```python
from build123d import *

# Parameters (mm, degrees)
SKETCH1_W           = 104
SKETCH1_H           = 104
BOSS_EXTRUDE1_DEPTH = 57.5
BOSS_EXTRUDE1_TAPER = 23
SKETCH2_R           = 25
CUT_EXTRUDE1_DEPTH  = 187.700294763
FILLET1_R           = 15
SKETCH3_R           = 35
CUT_EXTRUDE2_DEPTH  = 10
CUT_EXTRUDE3_START  = -10
SKETCH5_R           = 35
CUT_EXTRUDE3_DEPTH  = 10
SKETCH6_W           = 52
SKETCH6_H           = 52
CUT_EXTRUDE4_DEPTH  = 187.700294763
BOSS_EXTRUDE2_DEPTH = 10
FILLET2_R           = 5
CUT_EXTRUDE5_DEPTH  = 10


with BuildPart() as part:
    # Sketch1 → Boss-Extrude1 (new body)
    with BuildSketch(Plane(origin=(0, 0, 0), x_dir=(1, 0, 0), z_dir=(0, 1, 0))):
        with Locations((52, 52)):
            Rectangle(SKETCH1_W, SKETCH1_H)
    extrude(amount=BOSS_EXTRUDE1_DEPTH, taper=BOSS_EXTRUDE1_TAPER)

    # Mirror1: part across plane


with BuildPart() as part_1:
    add(part.part)
    add(part.part.mirror(Plane(origin=(0, 57.5, 0), x_dir=(0, 0, 1), z_dir=(0, -1, 0))))

    # Sketch2 → Cut-Extrude1 (cut, through all)
    with BuildSketch(Plane(origin=(0, 115, 0), x_dir=(1, 0, 0), z_dir=(0, 1, 0))):
        with Locations(Location((52, 52, 0), (0, 0, 270))):
            Circle(SKETCH2_R)
    extrude(amount=-CUT_EXTRUDE1_DEPTH, mode=Mode.SUBTRACT)

    # Fillet1
    # the kernel refuses this fillet: 15 mm, written as the material it adds along each edge
    with BuildSketch(Plane(origin=(24.407301932, 57.5, -95.510503676), x_dir=(-0.39073112848927455, -0.9205048534524399, 0), z_dir=(0, 0, 1))) as fillet1_piece_1_section:
        with BuildLine():
            CenterArc((FILLET1_R * 0.42447481621, -FILLET1_R), FILLET1_R, 90, 46)
            Line((-FILLET1_R * 0.294864984129, -FILLET1_R * 0.305341629541), (0, 0))
            Line((0, 0), (FILLET1_R * 0.42447481621, 0))
        make_face()
    fillet1_piece_1 = extrude(amount=87.021007352, mode=Mode.PRIVATE)
    fillet1_piece_1 = fillet1_piece_1 - Plane(origin=(24.407301932, 57.5, -8.111896271), x_dir=(0, -0.39073112848927466, -0.9205048534524399), z_dir=(-1, 0, 0)) * Cylinder(15, 200, mode=Mode.PRIVATE)
    fillet1_piece_1 = fillet1_piece_1 - Plane(origin=(24.407301932, 57.5, -95.888103729), x_dir=(0, -0.3907311284892748, 0.9205048534524398), z_dir=(1, 0, 0)) * Cylinder(15, 200, mode=Mode.PRIVATE)
    add(fillet1_piece_1)
    with BuildSketch(Plane(origin=(8.489496324, 57.5, -24.407301932), x_dir=(0, -0.9205048534524399, 0.39073112848927455), z_dir=(1, 0, 0))) as fillet1_piece_2_section:
        with BuildLine():
            CenterArc((FILLET1_R * 0.42447481621, -FILLET1_R), FILLET1_R, 90, 46)
            Line((-FILLET1_R * 0.294864984129, -FILLET1_R * 0.305341629541), (0, 0))
            Line((0, 0), (FILLET1_R * 0.42447481621, 0))
        make_face()
    fillet1_piece_2 = extrude(amount=87.021007352, mode=Mode.PRIVATE)
    fillet1_piece_2 = fillet1_piece_2 - Plane(origin=(95.888103729, 57.5, -24.407301932), x_dir=(-0.9205048534524398, -0.3907311284892748, 0), z_dir=(0, 0, 1)) * Cylinder(15, 200, mode=Mode.PRIVATE)
    fillet1_piece_2 = fillet1_piece_2 - Plane(origin=(8.111896271, 57.5, -24.407301932), x_dir=(0.9205048534524399, -0.39073112848927466, 0), z_dir=(0, 0, -1)) * Cylinder(15, 200, mode=Mode.PRIVATE)
    add(fillet1_piece_2)
    with BuildSketch(Plane(origin=(79.592698068, 57.5, -8.489496324), x_dir=(0.39073112848927455, -0.9205048534524399, 0), z_dir=(0, 0, -1))) as fillet1_piece_3_section:
        with BuildLine():
            CenterArc((FILLET1_R * 0.42447481621, -FILLET1_R), FILLET1_R, 90, 46)
            Line((-FILLET1_R * 0.294864984129, -FILLET1_R * 0.305341629541), (0, 0))
            Line((0, 0), (FILLET1_R * 0.42447481621, 0))
        make_face()
    fillet1_piece_3 = extrude(amount=87.021007352, mode=Mode.PRIVATE)
    fillet1_piece_3 = fillet1_piece_3 - Plane(origin=(79.592698068, 57.5, -8.111896271), x_dir=(0, -0.39073112848927466, -0.9205048534524399), z_dir=(-1, 0, 0)) * Cylinder(15, 200, mode=Mode.PRIVATE)
    fillet1_piece_3 = fillet1_piece_3 - Plane(origin=(79.592698068, 57.5, -95.888103729), x_dir=(0, -0.3907311284892748, 0.9205048534524398), z_dir=(1, 0, 0)) * Cylinder(15, 200, mode=Mode.PRIVATE)
    add(fillet1_piece_3)
    with BuildSketch(Plane(origin=(95.510503676, 57.5, -79.592698068), x_dir=(0, -0.9205048534524399, -0.39073112848927455), z_dir=(-1, 0, 0))) as fillet1_piece_4_section:
        with BuildLine():
            CenterArc((FILLET1_R * 0.42447481621, -FILLET1_R), FILLET1_R, 90, 46)
            Line((-FILLET1_R * 0.294864984129, -FILLET1_R * 0.305341629541), (0, 0))
            Line((0, 0), (FILLET1_R * 0.42447481621, 0))
        make_face()
    fillet1_piece_4 = extrude(amount=87.021007352, mode=Mode.PRIVATE)
    fillet1_piece_4 = fillet1_piece_4 - Plane(origin=(95.888103729, 57.5, -79.592698068), x_dir=(-0.9205048534524398, -0.3907311284892748, 0), z_dir=(0, 0, 1)) * Cylinder(15, 200, mode=Mode.PRIVATE)
    fillet1_piece_4 = fillet1_piece_4 - Plane(origin=(8.111896271, 57.5, -79.592698068), x_dir=(0.9205048534524399, -0.39073112848927466, 0), z_dir=(0, 0, -1)) * Cylinder(15, 200, mode=Mode.PRIVATE)
    add(fillet1_piece_4)

    # Sketch3 → Cut-Extrude2 (cut)
    with BuildSketch(Plane(origin=(0, 115, 0), x_dir=(1, 0, 0), z_dir=(0, 1, 0))):
        with Locations(Location((52, 52, 0), (0, 0, 270))):
            Circle(SKETCH3_R)
    extrude(amount=-CUT_EXTRUDE2_DEPTH, mode=Mode.SUBTRACT)

    # Sketch5 → Cut-Extrude3 (cut)
    with BuildSketch(Plane.XZ.offset(CUT_EXTRUDE3_START)):
        with Locations(Location((52, -52, 0), (0, 0, 90))):
            Circle(SKETCH5_R)
    extrude(amount=CUT_EXTRUDE3_DEPTH, mode=Mode.SUBTRACT)

    # Sketch6 → Cut-Extrude4 (cut, through all)
    with BuildSketch(Plane(origin=(0, 115, 0), x_dir=(1, 0, 0), z_dir=(0, 1, 0))):
        with Locations((78, 26)):
            Rectangle(SKETCH6_W, SKETCH6_H)
    extrude(amount=-CUT_EXTRUDE4_DEPTH, mode=Mode.SUBTRACT)

    # Sketch7 → Boss-Extrude2 (add)
    with BuildSketch(Plane(origin=(0, 115, 0), x_dir=(1, 0, 0), z_dir=(0, 1, 0))):
        Polygon((52, 17), (52, 0), (0, 0), (0, 104), (104, 104), (104, 52), (87, 52), (87, 55), (101, 55), (101, 101), (3, 101), (3, 3), (49, 3), (49, 17), align=None)
    extrude(amount=BOSS_EXTRUDE2_DEPTH)

    # Fillet2
    fillet2_edges = [part_1.edges().sort_by_distance(p)[0] for p in [
        (26, 115, -3),
        (0, 115, -52),
        (52, 115, -104),
        (104, 115, -78),
    ]]
    fillet(fillet2_edges, radius=FILLET2_R)

    # Sketch8 → Cut-Extrude5 (cut)
    with BuildSketch(Plane(origin=(0, 115, 0), x_dir=(1, 0, 0), z_dir=(0, 1, 0))):
        with BuildLine():
            Line((12.760046787, 95.4825939), (23.366648505, 84.875992182))
            ThreePointArc((23.366648505, 84.875992182), (23.366648505, 80.633351495), (19.124007818, 80.633351495))
            Line((19.124007818, 80.633351495), (8.5174061, 91.239953213))
            ThreePointArc((8.5174061, 91.239953213), (8.5174061, 95.4825939), (12.760046787, 95.4825939))
        make_face()
        with BuildLine():
            Line((12.760046787, 8.5174061), (23.366648505, 19.124007818))
            ThreePointArc((23.366648505, 19.124007818), (23.366648505, 23.366648505), (19.124007818, 23.366648505))
            Line((19.124007818, 23.366648505), (8.5174061, 12.760046787))
            ThreePointArc((8.5174061, 12.760046787), (8.5174061, 8.5174061), (12.760046787, 8.5174061))
        make_face()
        with BuildLine():
            Line((91.239953213, 95.4825939), (80.633351495, 84.875992182))
            ThreePointArc((80.633351495, 84.875992182), (80.633351495, 80.633351495), (84.875992182, 80.633351495))
            Line((84.875992182, 80.633351495), (95.4825939, 91.239953213))
            ThreePointArc((95.4825939, 91.239953213), (95.4825939, 95.4825939), (91.239953213, 95.4825939))
        make_face()
    extrude(amount=-CUT_EXTRUDE5_DEPTH, mode=Mode.SUBTRACT)


solid = part_1.part
```
Check sheet for the modelled part. Datum: model origin and axes. Units: mm. A direction names the side the tool comes from. Give positions to 0.01 mm unless a question says otherwise; leave off trailing zeros. Write each loop counter-clockwise with the first axis right and the second up, starting at its lowest first coordinate (ties: lowest second). Pieces come first, ordered by that corner, then holes. Notation, with made-up numbers: (45.5, 2.5) -> (66.5, 2.5) arc R20 cw to (66.5, 10.5) -> close; hole circle Ø4 at (15, 88). An arc over 180 degrees is marked (long way). Use CSV: the item, a comma, the result in double quotes. Start each with the question number.
Q1. Release check for a two-part mould opening along X. For faces 4 (the flat face through (17.99, 110.07, -13.75)), 5 (the flat face through (23, 0, -73)) record: +X half, -X half, draft (parallel to the pull), parting line (faces both ways), or undercut.
Q2. Scan lines: line 1 along Y through (x, z) = (50, -77); line 2 along Z through (x, y) = (31.5, 30); line 3 along X through (y, z) = (89, -64.5). Record each from-to range of solid material in increasing order.
Q3. Tool access check on faces 1 (the cylindrical face through (8.471, 110.07, -95.435)), 2 (the flat face through (50, 120, -17)), 3 (the flat face through (79, 62, -52)). Record the directions out of +Z, -Z, +X, -X, +Y, -Y that give a thin tool (end or side, any length) a straight path to the whole face; none if there is none.
Q4. Cross-section at A-A on y = 55. Enter the section's corners in (x, z).
Q5. Depth check by flat-ended pin: P1, Ø1, axis at x = 20.5, y = 33.5, coming from the -Z side; P2, Ø8.5, axis at x = 19.5, z = -16, coming from the +Y side; P3, Ø12, axis at x = 84.5, y = 77.5, coming from the -Z side. Enter the tip coordinate at first touch or a pass-through.
Working result:
1,face 4,"undercut"
1,face 5,"draft"
2,line 1,"y = 10 to 105"
2,line 2,"z = -91.27 to -66.31, -37.69 to -12.73"
2,line 3,"x = 11.04 to 30.35, 73.65 to 92.96"
3,face 1,"+Y"
3,face 2,"+X, +Y"
3,face 3,"+Z, +X, +Y, -Y"
4,outline,"(22.9, -81.1) -> (81.1, -81.1) -> (81.1, -52) -> (77, -52) arc R25 cw (long way) to (52, -27) -> (52, -22.9) -> (22.9, -22.9) -> close"
5,P1,"stops at z = -89.99"
5,P2,"stops at y = 115"
5,P3,"stops at z = -90.63"
